from build123d import *

# Parameters (mm, degrees)
SKETCH_R      = 2
PAD_DEPTH     = 2
SKETCH001_W   = 75
SKETCH001_H   = 44
SKETCH001_W_2 = 73
SKETCH001_H_2 = 42
PAD001_DEPTH  = 32
SKETCH002_R   = 6
PAD002_DEPTH  = 58
SKETCH003_R   = 2.5
POCKET_DEPTH  = 10


with BuildPart() as part:
    # Sketch → Pad (new body)
    with BuildSketch(Plane.XY):
        with BuildLine():
            Line((37.5, 22), (37.5, 7.5))
            Line((37.5, 7.5), (85, 7.5))
            Line((85, 7.5), (85, -7.5))
            Line((85, -7.5), (37.5, -7.5))
            Line((37.5, -7.5), (37.5, -22))
            Line((37.5, -22), (17.5, -22))
            Line((17.5, -22), (17.5, -31.527864))
            ThreePointArc((9.027864, -40), (17.742641, -40.242641), (17.5, -31.527864))
            Line((9.027864, -40), (-54.027864, -40))
            ThreePointArc((-62.5, -31.527864), (-62.742641, -40.242641), (-54.027864, -40))
            Line((-62.5, -31.527864), (-62.5, -7.5))
            Line((-62.5, -7.5), (-85, -7.5))
            Line((-85, -7.5), (-85, 7.5))
            Line((-85, 7.5), (-62.5, 7.5))
            Line((-62.5, 7.5), (-62.5, 31.527864))
            ThreePointArc((-54.027864, 40), (-62.742641, 40.242641), (-62.5, 31.527864))
            Line((-54.027864, 40), (9.027864, 40))
            ThreePointArc((17.5, 31.527864), (17.742641, 40.242641), (9.027864, 40))
            Line((17.5, 31.527864), (17.5, 22))
            Line((17.5, 22), (37.5, 22))
        make_face()
        with Locations((-72.5, 0)):
            Circle(SKETCH_R, mode=Mode.SUBTRACT)
        with Locations((72.5, 0)):
            Circle(SKETCH_R, mode=Mode.SUBTRACT)
        with BuildLine():
            Line((-37.5, 22), (9.5, 22))
            Line((9.5, 31.527864), (9.5, 22))
            ThreePointArc((9.027864, 32), (9.257359, 31.757359), (9.5, 31.527864))
            Line((-54.027864, 32), (9.027864, 32))
            ThreePointArc((-54.5, 31.527864), (-54.257359, 31.757359), (-54.027864, 32))
            Line((-54.5, 7.5), (-54.5, 31.527864))
            Line((-54.5, 7.5), (-37.5, 7.5))
            Line((-37.5, 7.5), (-37.5, 22))
        make_face(mode=Mode.SUBTRACT)
        with BuildLine():
            Line((-37.5, -22), (-37.5, -7.5))
            Line((-37.5, -7.5), (-54.5, -7.5))
            Line((-54.5, -31.527864), (-54.5, -7.5))
            ThreePointArc((-54.027864, -32), (-54.257359, -31.757359), (-54.5, -31.527864))
            Line((9.027864, -32), (-54.027864, -32))
            ThreePointArc((9.5, -31.527864), (9.257359, -31.757359), (9.027864, -32))
            Line((9.5, -22), (9.5, -31.527864))
            Line((9.5, -22), (-37.5, -22))
        make_face(mode=Mode.SUBTRACT)
    extrude(amount=PAD_DEPTH)

    # Sketch001 → Pad001 (join)
    with BuildSketch(Plane.XY):
        Rectangle(SKETCH001_W, SKETCH001_H)
        Rectangle(SKETCH001_W_2, SKETCH001_H_2, mode=Mode.SUBTRACT)
    extrude(amount=PAD001_DEPTH)

    # Sketch002 → Pad002 (join)
    with BuildSketch(Plane.XY):
        with Locations((-58.486508, 36)):
            Circle(SKETCH002_R)
        with Locations((13.513492, 36)):
            Circle(SKETCH002_R)
        with Locations((-58.486508, -36)):
            Circle(SKETCH002_R)
        with Locations((13.513492, -36)):
            Circle(SKETCH002_R)
    extrude(amount=PAD002_DEPTH)

    # Sketch003 (on Face43 of Pad002) → Pocket (cut)
    with BuildSketch(Plane.XY.offset(58)):
        with Locations((-58.5, 36)):
            Circle(SKETCH003_R)
        with Locations((-58.5, -36)):
            Circle(SKETCH003_R)
        with Locations((13.5, -36)):
            Circle(SKETCH003_R)
        with Locations((13.5, 36)):
            Circle(SKETCH003_R)
    extrude(amount=-POCKET_DEPTH, mode=Mode.SUBTRACT)


solid = part.part
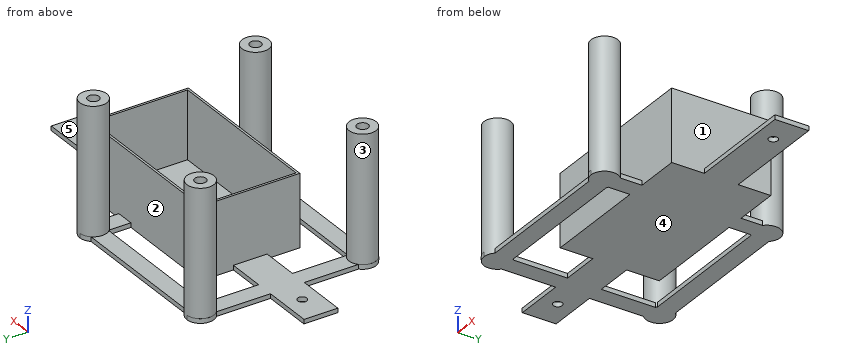
For this review, take the finished solid that the model builds, in its own axes (mm). Face numbers are marked on the shaded views. A direction names the side the tool comes from. Round coordinates to 2 decimals unless told otherwise and drop trailing zeros. Loops run counter-clockwise (first coordinate to the right, second up) from the corner with the lowest first, then second, coordinate; pieces in that order, holes last. Notation, with made-up numbers: (31, 4.5) - (39, 4.5) arc R25 ccw to (39, 17.5) - close; hole circle Ø4 at (88.25, -40). An arc over 180 degrees is marked (long way). Put each result on its own line as item: value. Start each with the question number.
1. Consider section C-C on x = -72.5. State the section outline as (y, z) points.
2. Mouldability with a two-part tool opening along Y and no side actions: class the marked faces 1 and 2 as +Y half, -Y half, draft (parallel to the pull), parting line (faces both ways), or undercut.
3. Consider section D-D on y = -16.5. State the section outline as (x, z) points.
4. For the marked faces 3, 4 and 5, list the 3-axis set-ups (+Z, -Z, +X, -X, +Y, -Y) from which the entire face can be reached by the end or side of a thin tool; tool diameter is ignored.
5. For probe 1 along Y at (x, z) = (-58.5, 52.5); probe 2 along X at (y, z) = (5, 15); probe 3 along Y at (x, z) = (-58, 54), list the stretches that pass through material, from the lowest coordinate up. Write a range as [from, to].
6. Insertion check: P1, Ø1.5, axis at x = -58, y = 35, coming from the +Z side; P2, Ø9.5, axis at y = 5, z = 17.5, coming from the -X side; P3, Ø4, axis at x = 0, z = 35, coming from the -Y side; P4, Ø0.6, axis at x = -26, z = 1, coming from the +Y side. Each pin has a flat end and moves straight along its axis. Give the tip position at first contact, or say it passes through.
7. Consider section A-A on z = 51. State the section outline as (x, y) points.
8. Consider section B-B on z = 17. State the section outline as (x, y) points, plus the area to 3 significant figures.
Result sheet:
1. outline: (-7.5, 0) - (-2, 0) - (-2, 2) - (-7.5, 2) - close; (2, 0) - (7.5, 0) - (7.5, 2) - (2, 2) - close
2. face 1: draft
2. face 2: undercut
3. outline: (-62.5, 0) - (-54.5, 0) - (-54.5, 2) - (-62.5, 2) - close; (-37.5, 0) - (37.5, 0) - (37.5, 32) - (36.5, 32) - (36.5, 2) - (-36.5, 2) - (-36.5, 32) - (-37.5, 32) - close
4. face 3: +Z
4. face 4: -Z, +X, -X, +Y, -Y
4. face 5: +Z, +X, +Y, -Y
5. probe 1: [-42, -38.5], [-33.5, -30], [30, 33.5], [38.5, 42]
5. probe 2: [-37.5, -36.5], [36.5, 37.5]
5. probe 3: [-41.98, -38.45], [-33.55, -30.02], [30.02, 33.55], [38.45, 41.98]
6. P1: z = 48
6. P2: x = -37.5
6. P3: through
6. P4: y = 40
7. outline: circle Ø12 at (-58.49, -36); circle Ø12 at (-58.49, 36); circle Ø12 at (13.51, -36); circle Ø12 at (13.51, 36); hole circle Ø5 at (-58.5, -36); hole circle Ø5 at (-58.5, 36); hole circle Ø5 at (13.5, -36); hole circle Ø5 at (13.5, 36)
8. outline: circle Ø12 at (-58.49, -36); circle Ø12 at (-58.49, 36); (-37.5, -22) - (37.5, -22) - (37.5, 22) - (-37.5, 22) - close; circle Ø12 at (13.51, -36); circle Ø12 at (13.51, 36); hole (-36.5, -21) - (36.5, -21) - (36.5, 21) - (-36.5, 21) - close
8. area: 686 mm^2
